Verification items for the finished model (mm, model axes). Give positions to 0.01 mm unless a question says otherwise; leave off trailing zeros. Write each loop counter-clockwise with the first axis right and the second up, starting at its lowest first coordinate (ties: lowest second). Pieces come first, ordered by that corner, then holes.
from build123d import *

# Parameters (mm, degrees)
SKETCH1_W           = 140
SKETCH1_H           = 100
BOSS_EXTRUDE1_DEPTH = 6.35
SKETCH2_R           = 12.705
SKETCH2_R_2         = 5
CUT_EXTRUDE1_DEPTH  = 10
SKETCH3_R           = 1.5875
CUT_EXTRUDE2_DEPTH  = 10


with BuildPart() as part:
    # Sketch1 → Boss-Extrude1 (new body)
    with BuildSketch(Plane(origin=(0, 0, 0), x_dir=(1, 0, 0), z_dir=(0, 1, 0))):
        with Locations((70, 50)):
            Rectangle(SKETCH1_W, SKETCH1_H)
    extrude(amount=BOSS_EXTRUDE1_DEPTH)

    # Sketch2 → Cut-Extrude1 (cut)
    with BuildSketch(Plane(origin=(0, 6.35, 0), x_dir=(1, 0, 0), z_dir=(0, 1, 0))):
        with Locations(Location((103.75, 30.514428415, 0), (0, 0, 270))):
            Circle(SKETCH2_R)
        with Locations(Location((92.5, 50, 0), (0, 0, 270))):
            Circle(SKETCH2_R_2)
    extrude(amount=-CUT_EXTRUDE1_DEPTH, mode=Mode.SUBTRACT)

    # Sketch3 → Cut-Extrude2 (cut)
    with BuildSketch(Plane(origin=(0, 6.35, 0), x_dir=(1, 0, 0), z_dir=(0, 1, 0))):
        with Locations(Location((8.85, 50, 0), (0, 0, 270))):
            Circle(SKETCH3_R)
        with Locations(Location((131.15, 50, 0), (0, 0, 270))):
            Circle(SKETCH3_R)
        with Locations(Location((75, 58, 0), (0, 0, 270))):
            Circle(SKETCH3_R)
        with Locations(Location((110, 58, 0), (0, 0, 270))):
            Circle(SKETCH3_R)
    extrude(amount=-CUT_EXTRUDE2_DEPTH, mode=Mode.SUBTRACT)


solid = part.part
Item 1: Sectioned sample at B-B on z = -50. Record the cut outline in (x, y), then the cut area to 3 significant figures.
Answer key:
outline: (0, 0) - (7.26, 0) - (7.26, 6.35) - (0, 6.35) - close; (10.44, 0) - (87.5, 0) - (87.5, 6.35) - (10.44, 6.35) - close; (97.5, 0) - (129.56, 0) - (129.56, 6.35) - (97.5, 6.35) - close; (132.74, 0) - (140, 0) - (140, 6.35) - (132.74, 6.35) - close
area: 785 mm2
Item 2: Release check for a two-part mould opening along Z. For faces 1 (the face through (69, 0, -51)), 2 (the face through (129.74, 3.22, -49.27)), 3 (the face through (69, 3, 0)) record: released by +Z, released by -Z, zero draft, split by the parting line, or undercut.
Answer key:
face 1: zero draft
face 2: undercut
face 3: released by +Z
Item 3: Scan lines: line 1 along X through (y, z) = (3.5, -58); line 2 along Z through (x, y) = (131, 5.5); line 3 along X through (y, z) = (4.25, -57). Record each from-to range of solid material in increasing order.
Answer key:
line 1: x = 0 to 73.41, 76.59 to 108.41, 111.59 to 140
line 2: z = -100 to -51.58, -48.42 to 0
line 3: x = 0 to 73.77, 76.23 to 108.77, 111.23 to 140
Item 4: Depth check by flat-ended pin: pin 1 (1.9 mm diameter, centred on x = 8.85, z = -50, fed in from -Y). Enter the tip coordinate at first touch or a pass-through.
Answer key:
pin 1: passes through
Item 5: Sectioned sample at D-D on x = 92.5. Record the cut outline in (y, z), then the cut area to 3 significant figures.
Answer key:
outline: (0, -100) - (6.35, -100) - (6.35, -55) - (0, -55) - close; (0, -45) - (6.35, -45) - (6.35, -36.42) - (0, -36.42) - close; (0, -24.61) - (6.35, -24.61) - (6.35, 0) - (0, 0) - close
area: 497 mm2
Item 6: Sectioned sample at C-C on x = 131.15. Record the cut outline in (y, z), then the cut area to 3 significant figures.
Answer key:
outline: (0, -100) - (6.35, -100) - (6.35, -51.59) - (0, -51.59) - close; (0, -48.41) - (6.35, -48.41) - (6.35, 0) - (0, 0) - close
area: 615 mm2
Item 7: Sectioned sample at A-A on y = 4.5. State how many separate pieces and enclosed holes the cut face has, then the cut area to 3 significant figures.
Answer key:
separate pieces: 1
enclosed holes: 6
area: 13,400 mm2
